from build123d import *

# Parameters (mm, degrees)
F2_R      = 25.9962792711
F3_DEPTH  = 1219.2
F4_R      = 26.4847844062
F5_DEPTH  = 1524
F6_R      = 36.4583411444
F7_DEPTH  = 1219.2
F8_W      = 1525.4385471344
F8_H      = 1222.8087186813
F9_DEPTH  = 25.4
F15_DEPTH = 27.77983


# Not quite as in the source:
# - the program builds the solid bodies; features that only make, move or delete a surface that nothing else refers to are left out


with BuildPart() as f3:
    # F2 (on Front) → F3 (new body)
    with BuildSketch(Plane.XZ):
        Circle(F2_R)
    extrude(amount=F3_DEPTH)

    # F4 (on Right) → F5 (join)
    with BuildSketch(Plane.YZ):
        with Locations((-1223.8247394562, 0)):
            Circle(F4_R)
    extrude(amount=F5_DEPTH)

    # F6 (on Front) → F7 (join)
    with BuildSketch(Plane.XZ):
        with Locations((1525.4992246628, 0)):
            Circle(F6_R)
    extrude(amount=F7_DEPTH)

    # F8 (on Top) → F9 (join)
    with BuildSketch(Plane.XY):
        with Locations((762.7192735672, -611.4043593407)):
            Rectangle(F8_W, F8_H)
    extrude(amount=F9_DEPTH)

    # F15 (add): a face of the model
    f15_faces = [f3.faces().sort_by_distance(p)[0] for p in [
        (752.4403971283, -608.161243113, 25.4),
    ]]
    extrude(f15_faces, amount=-F15_DEPTH)


solid = f3.part
Read the model definition and answer for the solid it produces. Units are mm, in the model's axes. A direction names the side the tool comes from. Coordinates: 2 decimals unless noted, no trailing zeros. Loops run counter-clockwise (first coordinate to the right, second up) from the corner with the lowest first, then second, coordinate; pieces in that order, holes last. Notation, with made-up numbers: (61, 72.5) -> (110, 72.5) arc R32 ccw to (110, 106.5) -> close; hole circle Ø8 at (14, 12). An arc over 180 degrees is marked (long way). Write item = value, one per line. Start each with the question number.
1) Given P1, Ø3, axis at y = -830.5, z = 22, coming from the -X side; P2, Ø12, axis at x = 1090, z = 24, coming from the -Y side; P3, Ø25, axis at y = -1238, z = 9.5, coming from the +X side, each flat-ended and moving along its own axis, determine where each tip first touches the part or whether it passes through.
2) The part is cut by section A-A, the plane x = 1310. Determine the outline of the cut face in (y, z), plus the area to 3 significant figures.
3) Find the intervals of material crossed by L1, parallel to X at y = -581, z = -2.5; L2, parallel to Z at x = 966, y = -117.5; L3, parallel to X at y = -126.5, z = -8, in increasing order. Write a range as from..to.
4) The mould has two halves that part along X. Classify faces 1 (the face through (0, -1231, 0)), 2 (the face through (1524, -1235, 0)), 3 (the face through (751.33, -1246.23, -14.12)): pulls with the +X half, pulls with the -X half, needs draft (parallel to the pull), parting line crosses it, or undercut.
5) The part is cut by section B-B, the plane y = -1167. Determine the outline of the cut face in (x, z).
6) For faces 4 (the face through (-21.48, -601.07, -14.64)), 5 (the face through (757, 0, 17)), 6 (the face through (747, -590, -2.38)), determine the directions among +Z, -Z, +X, -X, +Y, -Y from which every point of the face is accessible in a straight line to the end or side of a thin tool.
Result:
q1.P1 = -15.99
q1.P2 = -1243.25
q1.P3 = 1524
q2.outline = (-1216.32, 25.4) arc R26.48 ccw (long way) to (-1197.45, -2.38) -> (0, -2.38) -> (0, 25.4) -> close
q2.area = 35,600 mm²
q3.L1 = -25.88..25.88, 1489.13..1561.87
q3.L2 = -2.38..25.4
q3.L3 = -24.73..24.73, 1489.93..1561.07
q4.face_1 = pulls with the -X half
q4.face_2 = pulls with the +X half
q4.face_3 = undercut
q5.outline = (5.54, 25.4) arc R26 ccw (long way) to (25.89, -2.38) -> (1489.12, -2.38) arc R36.46 ccw (long way) to (1499.34, 25.4) -> close
q6.face_4 = +Y
q6.face_5 = +Z, -Z, +X, -X, +Y
q6.face_6 = -Z, +Y
